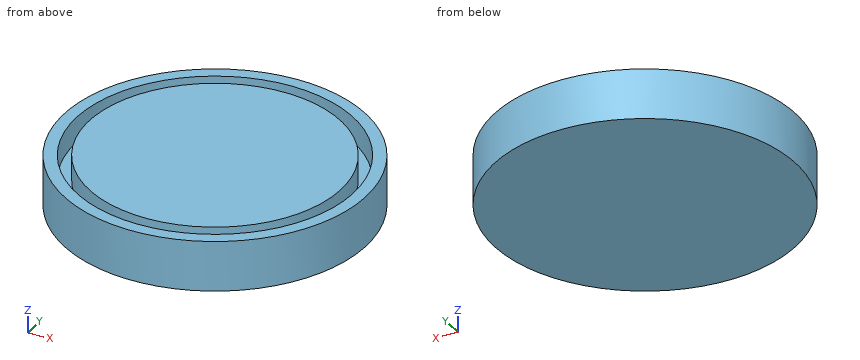
from build123d import *

# Parameters (mm, degrees)
F0_R      = 30
F0_R_2    = 27.5
F1_DEPTH  = 5
F2_DEPTH  = 10
F3_DEPTH  = 7.5
F4_R      = 30
F5_DEPTH  = 5
F6_R      = 30
F6_R_2    = 27.5
F7_DEPTH  = 2.5
F8_R      = 17.5
F9_DEPTH  = 3
F10_R     = 25
F11_DEPTH = 10


# Not quite as in the source:
# - a feature names something its author has since deleted; it is built from what else it names


with BuildPart() as f1:
    # F0 (on Top) → F1 (new body)
    with BuildSketch(Plane.XY):
        Circle(F0_R)
        Circle(F0_R_2, mode=Mode.SUBTRACT)
    extrude(amount=F1_DEPTH)

    # F0 (on Top) → F2 (join)
    with BuildSketch(Plane.XY):
        Circle(F0_R)
        Circle(F0_R_2, mode=Mode.SUBTRACT)
    extrude(amount=F2_DEPTH)

    # F0 (on Top) → F3 (join)
    with BuildSketch(Plane.XY):
        Circle(F0_R)
        Circle(F0_R_2, mode=Mode.SUBTRACT)
    extrude(amount=F3_DEPTH)

    # F4 (on Top) → F5 (join)
    with BuildSketch(Plane.XY):
        Circle(F4_R)
    extrude(amount=F5_DEPTH)

    # F6 (on Top) → F7 (join)
    with BuildSketch(Plane.XY):
        Circle(F6_R)
        Circle(F6_R_2, mode=Mode.SUBTRACT)
    extrude(amount=F7_DEPTH)

    # F8 (on Top) → F9 (join)
    with BuildSketch(Plane.XY):
        Circle(F8_R)
    extrude(amount=F9_DEPTH)

    # F10 (on Top) → F11 (join)
    with BuildSketch(Plane.XY):
        Circle(F10_R)
    extrude(amount=F11_DEPTH)


solid = f1.part
Read the model definition and answer for the solid it produces. Units are mm, in the model's axes. Give positions to 0.01 mm unless a question says otherwise; leave off trailing zeros. Write each loop counter-clockwise with the first axis right and the second up, starting at its lowest first coordinate (ties: lowest second). Pieces come first, ordered by that corner, then holes. Notation, with made-up numbers: M 63,-40 L 74,-40 A23 ccw 74,-28 Z; hole C 49.5,35 d9. An arc over 180 degrees is marked long. One line per item, written item: value. Start each with the question number.
(1) Find section A-A (z = 8.5). Determine the outline of the cut face in (x, y).
(2) Find section D-D (z = 1.75). Determine the outline of the cut face in (x, y), plus the area to 3 significant figures.
(3) Find section B-B (y = 0). Determine the outline of the cut face in (x, z), plus the area to 3 significant figures.
(4) Flat-ended cylindrical pins translate along their axes: pin 1 Ø1.5 at (y, z) = (-14.5, 8) entering from -X; pin 2 Ø1.5 at (x, z) = (5.5, 5.5) entering from -Y; pin 3 Ø2 at (y, z) = (20, 3) entering from -X. Find the tip coordinate at first contact, or state that the pin passes through.
(5) Find the intervals of material crossed by line 1 (Y direction, x = 0, z = 6.65); line 2 (X direction, y = -18, z = 9.5); line 3 (X direction, y = -13.5, z = 6.5), in increasing order.
Results below:
1. outline: C 0,0 d60; C 0,0 d50; hole C 0,0 d55
2. outline: C 0,0 d60
2. area: 2,830 mm^2
3. outline: M -30,0 L 30,0 L 30,10 L 27.5,10 L 27.5,5 L 25,5 L 25,10 L -25,10 L -25,5 L -27.5,5 L -27.5,10 L -30,10 Z
3. area: 575 mm^2
4. pin 1: stops at x = -26.66
4. pin 2: stops at y = -29.62
4. pin 3: stops at x = -23.22
5. line 1: y = -30 to -27.5, -25 to 25, 27.5 to 30
5. line 2: x = -24 to -20.79, -17.35 to 17.35, 20.79 to 24
5. line 3: x = -26.79 to -23.96, -21.04 to 21.04, 23.96 to 26.79
